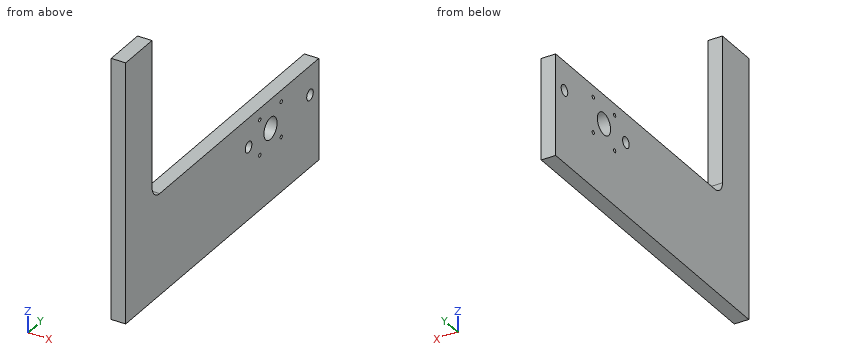
```python
from build123d import *

# Parameters (mm, degrees)
SKETCH1_R           = 4.7625
SKETCH1_R_2         = 9.525
SKETCH1_R_3         = 1.5875
BOSS_EXTRUDE1_DEPTH = 12.7


with BuildPart() as part:
    # Sketch1 → Boss-Extrude1 (new body)
    with BuildSketch(Plane(origin=(0, 0, 0), x_dir=(0, 0, -1), z_dir=(1, 0, 0))):
        with BuildLine():
            Line((0, 0), (0, 38.1))
            Line((0, 38.1), (128.5875, 38.1))
            ThreePointArc((128.5875, 38.1), (136.445224106, 41.354775894), (139.7, 49.2125))
            Line((139.7, 49.2125), (139.7, 279.4))
            Line((139.7, 279.4), (228.6, 279.4))
            Line((228.6, 279.4), (228.6, 0))
            Line((228.6, 0), (0, 0))
        make_face()
        with Locations((165.1, 266.7)):
            Circle(SKETCH1_R, mode=Mode.SUBTRACT)
        with Locations((165.1, 177.8)):
            Circle(SKETCH1_R, mode=Mode.SUBTRACT)
        with Locations((165.1, 209.55)):
            Circle(SKETCH1_R_2, mode=Mode.SUBTRACT)
        with Locations((180.599999988, 225.049999988)):
            Circle(SKETCH1_R_3, mode=Mode.SUBTRACT)
        with Locations((149.611999988, 225.049999988)):
            Circle(SKETCH1_R_3, mode=Mode.SUBTRACT)
        with Locations((180.599999988, 194.061999988)):
            Circle(SKETCH1_R_3, mode=Mode.SUBTRACT)
        with Locations((149.611999988, 194.061999988)):
            Circle(SKETCH1_R_3, mode=Mode.SUBTRACT)
    extrude(amount=BOSS_EXTRUDE1_DEPTH)


solid = part.part
```
Input: part model. Units: mm. Frame: model coordinates. Coordinates: 2 decimals unless noted, no trailing zeros. Order: outer loops, then holes, each group sorted by start corner. A loop starts at its lowest first (then second) coordinate and runs counter-clockwise, first axis right, second up. Notation, with made-up numbers: (78.25, 89.25) - (137.25, 89.25) arc R25 ccw to (137.25, 125.25) - close; hole circle Ø5 at (-17, -29.5). An arc over 180 degrees is marked (long way). Put each result on its own line as item: value.
1. Cut plane C-C on y = 209.55. Return the cut outline in (x, z) (3 decimals), then the cut area to 3 significant figures.
Report:
outline: (0, -228.6) - (12.7, -228.6) - (12.7, -174.625) - (0, -174.625) - close; (0, -155.575) - (12.7, -155.575) - (12.7, -139.7) - (0, -139.7) - close
area: 887 mm2
2. Cut plane B-B on z = -165.1. Return the cut outline in (x, y) (1 decimal), then the cut area to 3 significant figures.
Report:
outline: (0, 0) - (12.7, 0) - (12.7, 173) - (0, 173) - close; (0, 182.6) - (12.7, 182.6) - (12.7, 200) - (0, 200) - close; (0, 219.1) - (12.7, 219.1) - (12.7, 261.9) - (0, 261.9) - close; (0, 271.5) - (12.7, 271.5) - (12.7, 279.4) - (0, 279.4) - close
area: 3,060 mm2
3. Cut plane A-A on y = 177.8. Return the cut outline in (x, z).
Report:
outline: (0, -228.6) - (12.7, -228.6) - (12.7, -169.86) - (0, -169.86) - close; (0, -160.34) - (12.7, -160.34) - (12.7, -139.7) - (0, -139.7) - close
4. Contact query for flat-ended pins moving along their axis: pin 1 Ø4 at (x, y) = (2, 95.5) entering from +Z; pin 2 Ø6.5 at (x, z) = (3, -82) entering from +Y. Output: stop coordinate, or through.
Report:
pin 1: stops at z = -139.7
pin 2: stops at y = 38.1
5. Line query: line 1 along Z through (x, y) = (7.75, 225.05); line 2 along Y through (x, z) = (7, -165.1) (1 decimal); line 3 along Z through (x, y) = (3.25, 266.7). Output: solid intervals per line, ascending.
Report:
line 1: z = -228.6 to -182.19, -179.01 to -151.2, -148.02 to -139.7
line 2: y = 0 to 173, 182.6 to 200, 219.1 to 261.9, 271.5 to 279.4
line 3: z = -228.6 to -169.86, -160.34 to -139.7
6. Cut plane D-D on x = 3.25. State how many separate pieces and enclosed holes the cut face has, then the cut area to 3 significant figures.
Report:
separate pieces: 1
enclosed holes: 7
area: 29,700 mm2
